from build123d import *

# Parameters (mm, degrees)
SKETCH1_W               = 55
SKETCH1_H               = 80
BOSS_EXTRUDE1_DEPTH     = 10
SKETCH6_R               = 1.65
CUT_EXTRUDE2_DEPTH      = 55
LPATTERN1_COUNT         = 3
LPATTERN1_PITCH         = 25
MIRROR3_COPY_1_SKETCH_R = 1.65
MIRROR3_COPY_1_DEPTH    = 55
MIRROR3_COPY_2_SKETCH_R = 1.65
MIRROR3_COPY_2_DEPTH    = 55
SKETCH8_W               = 8
SKETCH8_H               = 55
BOSS_EXTRUDE3_DEPTH     = 65
FILLET3_R               = 5
SKETCH9_R               = 4.25
CUT_EXTRUDE3_DEPTH      = 32.5
CUT_EXTRUDE5_START      = -5
SKETCH11_R              = 3
CUT_EXTRUDE5_DEPTH      = 71
LPATTERN2_COUNT         = 3
LPATTERN2_PITCH         = 25
MIRROR4_START           = -5
MIRROR4_COPY_1_SKETCH_R = 3
MIRROR4_COPY_1_DEPTH    = 71
MIRROR4_COPY_2_SKETCH_R = 3
MIRROR4_COPY_2_DEPTH    = 71
CUT_EXTRUDE6_DEPTH      = 10
SKETCH13_R              = 4.15
BOSS_EXTRUDE4_DEPTH     = 23.5
SKETCH14_R              = 4.15
CUT_EXTRUDE7_DEPTH      = 20


with BuildPart() as part:
    # Sketch1 → Boss-Extrude1 (new body)
    with BuildSketch(Plane(origin=(0, 0, 0), x_dir=(1, 0, 0), z_dir=(0, 1, 0))):
        Rectangle(SKETCH1_W, SKETCH1_H)
    extrude(amount=BOSS_EXTRUDE1_DEPTH)

    # Sketch6 → Cut-Extrude2 (cut)
    with BuildSketch(Plane(origin=(0, 10, 0), x_dir=(1, 0, 0), z_dir=(0, 1, 0))):
        with Locations((-12.5, -25)):
            Circle(SKETCH6_R)
    cut_extrude2 = extrude(amount=-CUT_EXTRUDE2_DEPTH, mode=Mode.SUBTRACT)

    # LPattern1: Cut-Extrude2 ×3
    with Locations(*[(0, 0, -i * LPATTERN1_PITCH) for i in range(1, LPATTERN1_COUNT)]):
        add(cut_extrude2, mode=Mode.SUBTRACT)

    # Mirror3: Cut-Extrude2 across plane
    add(cut_extrude2.mirror(Plane(origin=(0, 0, 0), x_dir=(0, 0, 1), z_dir=(1, 0, 0))), mode=Mode.SUBTRACT)

    # Mirror3 copy 1 sketch → Mirror3 copy 1 (cut)
    with BuildSketch(Plane(origin=(0, 10, -25), x_dir=(-1, 0, 0), z_dir=(0, 1, 0))):
        with Locations((-12.5, 25)):
            Circle(MIRROR3_COPY_1_SKETCH_R)
    extrude(amount=-MIRROR3_COPY_1_DEPTH, mode=Mode.SUBTRACT)

    # Mirror3 copy 2 sketch → Mirror3 copy 2 (cut)
    with BuildSketch(Plane(origin=(0, 10, -50), x_dir=(-1, 0, 0), z_dir=(0, 1, 0))):
        with Locations((-12.5, 25)):
            Circle(MIRROR3_COPY_2_SKETCH_R)
    extrude(amount=-MIRROR3_COPY_2_DEPTH, mode=Mode.SUBTRACT)

    # Sketch8 → Boss-Extrude3 (add)
    with BuildSketch(Plane(origin=(0, 10, 0), x_dir=(1, 0, 0), z_dir=(0, 1, 0))):
        Rectangle(SKETCH8_W, SKETCH8_H)
    extrude(amount=BOSS_EXTRUDE3_DEPTH)

    # Fillet3
    fillet3_edges = [part.edges().sort_by_distance(p)[0] for p in [
        (4, 10, 0),
        (0, 10, -27.5),
        (-4, 10, 0),
        (0, 10, 27.5),
        (0, 75, -27.5),
        (0, 75, 27.5),
        (-27.5, 5, -40),
        (27.5, 5, -40),
    ]]
    fillet(fillet3_edges, radius=FILLET3_R)

    # Sketch9 → Cut-Extrude3 (cut, through all)
    with BuildSketch(Plane.ZY.offset(4)):
        with Locations((0, 50)):
            Circle(SKETCH9_R)
    extrude(amount=-CUT_EXTRUDE3_DEPTH, mode=Mode.SUBTRACT)

    # Sketch11 → Cut-Extrude5 (cut)
    with BuildSketch(Plane(origin=(0, 10, 0), x_dir=(1, 0, 0), z_dir=(0, 1, 0)).offset(CUT_EXTRUDE5_START)):
        with Locations((-12.5, -25)):
            Circle(SKETCH11_R)
    cut_extrude5 = extrude(amount=CUT_EXTRUDE5_DEPTH, mode=Mode.SUBTRACT)

    # LPattern2: Cut-Extrude5 ×3
    with Locations(*[(0, 0, -i * LPATTERN2_PITCH) for i in range(1, LPATTERN2_COUNT)]):
        add(cut_extrude5, mode=Mode.SUBTRACT)

    # Mirror4: Cut-Extrude5 across plane
    add(cut_extrude5.mirror(Plane(origin=(0, 0, 0), x_dir=(0, 0, 1), z_dir=(1, 0, 0))), mode=Mode.SUBTRACT)

    # Mirror4 copy 1 sketch → Mirror4 copy 1 (cut)
    with BuildSketch(Plane(origin=(0, 10, -25), x_dir=(-1, 0, 0), z_dir=(0, 1, 0)).offset(MIRROR4_START)):
        with Locations((-12.5, 25)):
            Circle(MIRROR4_COPY_1_SKETCH_R)
    extrude(amount=MIRROR4_COPY_1_DEPTH, mode=Mode.SUBTRACT)

    # Mirror4 copy 2 sketch → Mirror4 copy 2 (cut)
    with BuildSketch(Plane(origin=(0, 10, -50), x_dir=(-1, 0, 0), z_dir=(0, 1, 0)).offset(MIRROR4_START)):
        with Locations((-12.5, 25)):
            Circle(MIRROR4_COPY_2_SKETCH_R)
    extrude(amount=MIRROR4_COPY_2_DEPTH, mode=Mode.SUBTRACT)

    # Sketch12 → Cut-Extrude6 (cut)
    with BuildSketch(Plane(origin=(0, 10, 0), x_dir=(1, 0, 0), z_dir=(0, 1, 0))):
        Polygon((12.5, -37), (-38.055736231, -37), (-38.055736231, -44.287300659), (40.369344369, -44.287300659), (40.369344369, -37), align=None)
    extrude(amount=-CUT_EXTRUDE6_DEPTH, mode=Mode.SUBTRACT)

    # Sketch13 → Boss-Extrude4 (add)
    with BuildSketch(Plane.ZY.offset(4)):
        with BuildLine():
            Line((-7.35, 25), (-7.35, 0))
            Line((-7.35, 0), (7.35, 0))
            Line((7.35, 0), (7.35, 25))
            ThreePointArc((7.35, 25), (0, 32.35), (-7.35, 25))
        make_face()
        with Locations((0, 25)):
            Circle(SKETCH13_R, mode=Mode.SUBTRACT)
    extrude(amount=BOSS_EXTRUDE4_DEPTH)

    # Sketch14 → Cut-Extrude7 (cut)
    with BuildSketch(Plane.ZY.offset(4)):
        with Locations((0, 25)):
            Circle(SKETCH14_R)
    extrude(amount=-CUT_EXTRUDE7_DEPTH, mode=Mode.SUBTRACT)


solid = part.part
Model file for the job. Use its own axes, mm. A direction names the side the tool comes from. Give positions to 0.01 mm unless a question says otherwise; leave off trailing zeros. Loops run counter-clockwise (first coordinate to the right, second up) from the corner with the lowest first, then second, coordinate; pieces in that order, holes last. Notation, with made-up numbers: (-29, 74) -> (17, 74) arc R22 cw to (17, 93) -> close; hole circle Ø9 at (67, 75.25). An arc over 180 degrees is marked (long way). Use a Markdown table: item, result. Add a question column.
(1) Slice it at D-D on x = 0. List the corners of the cut face in (y, z).
(2) Drop flat-ended pins along their axis: pin 1 Ø12 at (x, z) = (5.5, 28.5) entering from +Y; pin 2 Ø11 at (y, z) = (50, 0) entering from +X; pin 3 Ø5.5 at (x, z) = (-12.5, -25) entering from +Y. Give the stop position or say it passes through.
(3) Slice it at B-B on y = 50. List the corners of the cut face in (x, z).
(4) Tool access for faces 1 (the flat face through (4, 45, 0)), 2 (the flat face through (0, 42, 27.5)), 3 (the flat face through (11, 5, 26)): list every direction of +Z, -Z, +X, -X, +Y, -Y with a clear straight run to the whole face (end or side of a thin tool).
(5) Mould opens along Z. For faces 4 (the cylindrical face through (-15.59, 32.35, 0.16)), 5 (the flat face through (-16, 17, 7.35)), 6 (the flat face through (-11, 5, 26)) say: +Z half, -Z half, draft (parallel to the pull), parting line (faces both ways), or undercut.
(6) Slice it at C-C on x = -12.5. List the corners of the cut face in (y, z), and give its area (3 significant figures).
(7) Wall check: line 1 along X through (y, z) = (7.9, -25); line 2 along Y through (x, z) = (-2, 0); line 3 along Z through (x, y) = (-12.5, 3.6). Give the ranges that are in metal, low to high.
(8) Slice it at A-A on z = 0. List the corners of the cut face in (x, y).
Filled sheet:
| question | item | result |
|---|---|---|
| 1 | outline | (0, -40) -> (10, -40) -> (10, -32.5) arc R5 cw to (15, -27.5) -> (70, -27.5) arc R5 ccw to (75, -22.5) -> (75, 22.5) arc R5 ccw to (70, 27.5) -> (15, 27.5) arc R5 cw to (10, 32.5) -> (10, 37) -> (0, 37) -> close; hole circle Ø8.3 at (25, 0); hole circle Ø8.5 at (50, 0) |
| 2 | pin 1 | y = 75 |
| 2 | pin 2 | x = 4 |
| 2 | pin 3 | y = 5 |
| 3 | outline | (-4, -27.5) -> (4, -27.5) -> (4, -4.25) -> (-4, -4.25) -> close; (-4, 4.25) -> (4, 4.25) -> (4, 27.5) -> (-4, 27.5) -> close |
| 4 | face 1 | +Z, -Z, +X, +Y |
| 4 | face 2 | +Z, +X, -X, +Y |
| 4 | face 3 | +Y |
| 5 | face 4 | parting line |
| 5 | face 5 | +Z half |
| 5 | face 6 | undercut |
| 6 | outline | (0, -40) -> (10, -40) -> (10, -28) -> (5, -28) -> (5, -26.65) -> (0, -26.65) -> close; (0, -23.35) -> (5, -23.35) -> (5, -22) -> (10, -22) -> (10, -7.35) -> (25, -7.35) arc R7.35 ccw to (25, 7.35) -> (10, 7.35) -> (10, 22) -> (5, 22) -> (5, 23.35) -> (0, 23.35) -> close; (0, 26.65) -> (5, 26.65) -> (5, 28) -> (10, 28) -> (10, 37) -> (0, 37) -> close; hole circle Ø8.3 at (25, 0) |
| 6 | area | 928 mm2 |
| 7 | line 1 | -27.5 to -15.5, -9.5 to 9.5, 15.5 to 27.5 |
| 7 | line 2 | 0 to 20.85, 29.15 to 45.75, 54.25 to 75 |
| 7 | line 3 | -40 to -26.65, -23.35 to 23.35, 26.65 to 37 |
| 8 | outline | (-27.5, 0) -> (10.85, 0) -> (10.85, 5) -> (9.5, 5) -> (9.5, 10) -> (9, 10) arc R5 cw to (4, 15) -> (4, 20.85) -> (-27.5, 20.85) -> close; (-27.5, 29.15) -> (4, 29.15) -> (4, 45.75) -> (-4, 45.75) -> (-4, 32.35) -> (-27.5, 32.35) -> close; (-4, 54.25) -> (4, 54.25) -> (4, 75) -> (-4, 75) -> close; (14.15, 0) -> (27.5, 0) -> (27.5, 10) -> (15.5, 10) -> (15.5, 5) -> (14.15, 5) -> close |
